Verification items for the finished model (mm, model axes). A direction names the side the tool comes from. Give positions to 0.01 mm unless a question says otherwise; leave off trailing zeros. Order: outer loops, then holes, each group sorted by start corner. A loop starts at its lowest first (then second) coordinate and runs counter-clockwise, first axis right, second up. Notation, with made-up numbers: (73, 52) - (132, 52) arc R22 ccw to (132, 80) - close; hole circle Ø2 at (0.5, -23.5). An arc over 180 degrees is marked (long way). Answer as a JSON object with one key per item and string values. Group by question number.
(1) Section check A-A (y = -13). Record the boundary of the cut face in (x, z), then the cut area to 3 significant figures.
(2) Thickness scan on line 1 (X direction, y = 17, z = 175); line 2 (X direction, y = 21.5, z = 77). Record the ranges inside material, lowest first.
(3) Access from +Z, -Z, +X, -X, +Y, -Y to the whole of each face (thin tool, end or side, straight path). Record for faces 1 (the face through (0, -23, 296)), 2 (the face through (0, -25, 296)).
(4) Section check C-C (z = 82). Record the boundary of the cut face in (x, y), then the cut area to 3 significant figures.
(5) Mould release check, pull along Y, two halves, no side actions. Record for faces 3 (the face through (-23, 0, 296)), 4 (the face through (25, 0, 296)), 5 (the face through (0, 25, 296)): +Y half, -Y half, draft (parallel to the pull), parting line (faces both ways), or undercut.
Autodesk Inventor part; units mm, degrees
ref_plane "Start Plane" through (0, 0, 25) normal (0, 0, 1) x (1, 0, 0)
ref_plane "End Plane" through (0, 0, 575.0026) normal (0, 0, 1) x (1, 0, 0)
ref_plane "Work Plane4" through (-1920, 21, 575.0026) normal (0, 0, 1) x (1, 0, 0)
ref_plane "Start Plane" through (0, 0, 25) normal (0, 0, 1) x (1, 0, 0)
ref_plane "End Plane" through (0, 0, 575.0026) normal (0, 0, 1) x (1, 0, 0)
sketch "Sketch" plane through (0, 0, 0) normal (0, 0, 1) x (1, 0, 0)
  line L0 (-25, -21) -> (-25, 21)
  line L1 (-21, 25) -> (21, 25)
  line L2 (25, 21) -> (25, -21)
  line L3 (21, -25) -> (-21, -25)
  arc A0 (-25, -21) -> (-21, -25) centre (-21, -21) ccw
  arc A1 (25, 21) -> (21, 25) centre (21, 21) ccw
  arc A2 (-21, 25) -> (-25, 21) centre (-21, 21) ccw
  arc A3 (21, -25) -> (25, -21) centre (21, -21) ccw
  arc A4 (-21, 23) -> (-23, 21) centre (-21, 21) ccw
  line L4 (-21, 23) -> (21, 23)
  arc A5 (23, 21) -> (21, 23) centre (21, 21) ccw
  line L5 (23, 21) -> (23, -21)
  arc A6 (21, -23) -> (23, -21) centre (21, -21) ccw
  line L6 (21, -23) -> (-21, -23)
  arc A7 (-23, -21) -> (-21, -23) centre (-21, -21) ccw
  line L7 (-23, -21) -> (-23, 21)
  line L8 (0, 36.1598) -> (0, -36.1598) construction
  line L9 (-36.1598, 0) -> (36.1598, 0) construction
  dimension "d7" = 4
  dimension "d9" = 50
  dimension "d11" = 50
  dimension "d12" = 2
  dimension "d15" = 25
  dimension "d16" = 25
extrude "Body" add sketch "Sketch" along normal up to surface (550.0026 mm away) from surface at 25
sketch "Sketch3" plane through (0, 0, 0) normal (0, 0, 1) x (1, 0, 0)
  line L0 (0, 0) -> (10, 0)
ref_plane "Work Plane3" through (0, 0, 0) normal (0, -1, 0) x (1, 0, 0)
sketch "Sketch4" plane through (0, 0, 0) normal (0, -1, 0) x (1, 0, 0)
  line L0 (-2, 25) -> (12, 25)
  line L1 (-2, 575.0026) -> (12, 575.0026)
  dimension "d18" = 550.0026
ref_plane "Work Plane4" through (-1920, 21, 575.0026) normal (0, 0, 1) x (1, 0, 0)
split "Split1" plane through (-1920, 21, 575.0026) removes the side toward (0, 0, 1)
ref_plane "Work Plane5" through (392.5, 21, 25) normal (0, 0, -1) x (-1, 0, 0)
split "Split2" plane through (392.5, 21, 25) removes the side toward (0, 0, -1)
equation "\"d7\" = G_IR"
equation "\"d9\" = G_W"
equation "\"d11\" = G_H"
equation "\"d12\" = G_T"
equation "\"d15\" = 0.5 * d9"
equation "\"d16\" = 0.5 * d11"
equation "\"d3\" = G_L"
equation "\"G_W\" = 50"
equation "\"G_H\" = 50"
equation "\"G_T\" = 2"
equation "\"G_IR\" = 4"
equation "\"G_L\" = d18"
equation "\"G_OFFSET_START\" = -25"
equation "\"G_OFFSET_END\" = -25"
equation "\"d13\" = -G_OFFSET_START"
equation "\"d14\" = G_OFFSET_END + B_L"
equation "\"B_L\" = 600.0026"
properties part number "ISO 10799-2 - 50x50x2 - 550"
Solutions:
{
 "1": {"outline": "(-25, 25) - (-23, 25) - (-23, 575) - (-25, 575) - close; (23, 25) - (25, 25) - (25, 575) - (23, 575) - close", "area": "2,200 mm2"},
 "2": {"line 1": "x = -25 to -23, 23 to 25", "line 2": "x = -24.97 to -22.94, 22.94 to 24.97"},
 "3": {"face 1": "+Z, -Z", "face 2": "+Z, -Z, +X, -X, -Y"},
 "4": {"outline": "(-25, -21) arc R4 ccw to (-21, -25) - (21, -25) arc R4 ccw to (25, -21) - (25, 21) arc R4 ccw to (21, 25) - (-21, 25) arc R4 ccw to (-25, 21) - close; hole (-23, -21) arc R2 ccw to (-21, -23) - (21, -23) arc R2 ccw to (23, -21) - (23, 21) arc R2 ccw to (21, 23) - (-21, 23) arc R2 ccw to (-23, 21) - close", "area": "374 mm2"},
 "5": {"face 3": "undercut", "face 4": "draft", "face 5": "+Y half"}
}
